Source: CAD feature listing. Evaluate the final solid. Frame: model axes, mm. Coordinates: 2 decimals unless noted, no trailing zeros. Order: outer loops, then holes, each group sorted by start corner. A loop starts at its lowest first (then second) coordinate and runs counter-clockwise, first axis right, second up.
Autodesk Inventor part; units mm, degrees
ref_plane "YZ Plane" through (0, 0, 0) normal (1, 0, 0) x (0, 1, 0)
ref_plane "XZ Plane" through (0, 0, 0) normal (0, 1, 0) x (-1, 0, 0)
ref_plane "XY Plane" through (0, 0, 0) normal (0, 0, 1) x (1, 0, 0)
sketch "Boceto1" plane through (0, 0, 0) normal (0, 0, 1) x (1, 0, 0)
  line L0 (0, 0) -> (0, 210)
  line L1 (0, 210) -> (450, 210)
  line L2 (450, 210) -> (450, 0)
  line L3 (450, 0) -> (0, 0)
  line L4 (0, 210) -> (5, 210)
  line L5 (5, 205) -> (50, 205)
  line L6 (50, 205) -> (50, 202)
  line L7 (5, 205) -> (5, 174.29)
  line L8 (5, 174.29) -> (8, 174.29)
  line L9 (8, 174.29) -> (8, 202)
  line L10 (8, 202) -> (50, 202)
  line L11 (0, 0) -> (5, 0)
  line L12 (0, 0) -> (5, 0)
  line L13 (5, 5) -> (50, 5)
  line L14 (5, 5) -> (5, 35.71)
  line L15 (5, 35.71) -> (8, 35.71)
  line L16 (50, 5) -> (50, 8)
  line L17 (8, 35.71) -> (8, 8)
  line L18 (8, 8) -> (50, 8)
  line L19 (450, 0) -> (445, 0)
  line L20 (445, 5) -> (445, 35.71)
  line L21 (445, 35.71) -> (442, 35.71)
  line L22 (445, 5) -> (400, 5)
  line L23 (400, 5) -> (400, 8)
  line L24 (400, 8) -> (442, 8)
  line L25 (442, 8) -> (442, 35.71)
  line L26 (450, 210) -> (445, 210)
  line L27 (445, 205) -> (400, 205)
  line L28 (445, 205) -> (445, 174.29)
  line L29 (445, 174.29) -> (442, 174.29)
  line L30 (400, 205) -> (400, 202)
  line L31 (400, 202) -> (442, 202)
  line L32 (442, 202) -> (442, 174.29)
  line L33 (5, 63.43) -> (5, 91.14)
  line L34 (5, 91.14) -> (8, 91.14)
  line L35 (8, 91.14) -> (8, 63.43)
  line L36 (8, 63.43) -> (5, 63.43)
  line L37 (5, 118.86) -> (5, 146.57)
  line L38 (5, 118.86) -> (8, 118.86)
  line L39 (8, 118.86) -> (8, 146.57)
  line L40 (8, 146.57) -> (5, 146.57)
  line L41 (445, 63.43) -> (445, 91.14)
  line L42 (445, 63.43) -> (442, 63.43)
  line L43 (442, 63.43) -> (442, 91.14)
  line L44 (442, 91.14) -> (445, 91.14)
  line L45 (445, 118.86) -> (442, 118.86)
  line L46 (442, 118.86) -> (442, 146.57)
  line L47 (442, 146.57) -> (445, 146.57)
  line L48 (445, 146.57) -> (445, 118.86)
  line L49 (350, 205) -> (300, 205)
  line L50 (300, 205) -> (300, 202)
  line L51 (300, 202) -> (350, 202)
  line L52 (350, 202) -> (350, 205)
  line L53 (250, 205) -> (200, 205)
  line L54 (200, 205) -> (200, 202)
  line L55 (200, 202) -> (250, 202)
  line L56 (250, 202) -> (250, 205)
  line L57 (150, 205) -> (100, 205)
  line L58 (100, 205) -> (100, 202)
  line L59 (100, 202) -> (150, 202)
  line L60 (150, 202) -> (150, 205)
  line L61 (350, 8) -> (300, 8)
  line L62 (300, 8) -> (300, 5)
  line L63 (300, 5) -> (350, 5)
  line L64 (350, 5) -> (350, 8)
  line L65 (250, 8) -> (200, 8)
  line L66 (200, 8) -> (200, 5)
  line L67 (200, 5) -> (250, 5)
  line L68 (250, 5) -> (250, 8)
  line L69 (150, 8) -> (100, 8)
  line L70 (100, 8) -> (100, 5)
  line L71 (100, 5) -> (150, 5)
  line L72 (150, 5) -> (150, 8)
  point P0 (450, 30)
  dimension "d8" = 210
  dimension "d9" = 210
  dimension "d10" = 5
  dimension "d11" = 27.72
  dimension "d12" = 5
  dimension "d13" = 5
  dimension "d14" = 450
  dimension "d15" = 5
  dimension "d16" = 5
  dimension "d17" = 5
  dimension "d18" = 45
  dimension "d19" = 30.71
  dimension "d20" = 3
  dimension "d21" = 3
  dimension "d22" = 30.71
  dimension "d23" = 45
  dimension "d24" = 3
  dimension "d25" = 3
  dimension "d26" = 5
  dimension "d27" = 5
  dimension "d29" = 5
  dimension "d30" = 30.71
  dimension "d31" = 45
  dimension "d32" = 5
  dimension "d33" = 3
  dimension "d34" = 3
  dimension "d35" = 5
  dimension "d36" = 5
  dimension "d37" = 45
  dimension "d38" = 30.71
  dimension "d39" = 3
  dimension "d40" = 3
  dimension "d41" = 50
  dimension "d42" = 5
  dimension "d43" = 5
  dimension "d44" = 5
  dimension "d45" = 3
  dimension "d46" = 3
sketch "Boceto2" plane through (0, 0, 0) normal (0, 0, 1) x (1, 0, 0)
  line L0 (449.8604, 0) -> (282.2704, 0)
  circle A0 centre (282.2704, 105) radius 80
  point P0 (0, 0)
extrude "Extrusión1" add sketch "Boceto1" along normal blind 3
extrude "Extrusión2" cut sketch "Boceto2" along normal blind 3
properties part number "Pieza agujero" material "Madera (nogal)"
Q1. Pull-direction query (Y, two-part tool) for faces 1 (the cylindrical face through (358.576, 80.97, 1.479)), 2 (the flat face through (172, 106, 3)); classes: pulls with the +Y half, pulls with the -Y half, needs draft (parallel to the pull), parting line crosses it, or undercut.
Solutions:
face 1: undercut
face 2: needs draft
Q2. Material intervals for line 1 along X through (y, z) = (194, 0.3); line 2 along Y through (x, z) = (405.5, 2.35); line 3 along Y through (x, z) = (247, 2.4), sorted ascending.
Solutions:
line 1: x = 0 to 5, 8 to 442, 445 to 450
line 2: y = 0 to 5, 8 to 202, 205 to 210
line 3: y = 0 to 5, 8 to 33.19, 176.81 to 202, 205 to 210
Q3. Section query A-A on x = 404.5. Output: boundary loops of the cut face in (y, z).
Solutions:
outline: (0, 0) - (5, 0) - (5, 3) - (0, 3) - close; (8, 0) - (202, 0) - (202, 3) - (8, 3) - close; (205, 0) - (210, 0) - (210, 3) - (205, 3) - close
Q4. Section query B-B on y = 105. Output: boundary loops of the cut face in (x, z), plus the area to 3 significant figures.
Solutions:
outline: (0, 0) - (202.27, 0) - (202.27, 3) - (0, 3) - close; (362.27, 0) - (450, 0) - (450, 3) - (362.27, 3) - close
area: 870 mm2
Q5. Section query C-C on y = 126. Output: boundary loops of the cut face in (x, z).
Solutions:
outline: (0, 0) - (5, 0) - (5, 3) - (0, 3) - close; (8, 0) - (205.08, 0) - (205.08, 3) - (8, 3) - close; (359.46, 0) - (442, 0) - (442, 3) - (359.46, 3) - close; (445, 0) - (450, 0) - (450, 3) - (445, 3) - close
Q6. Section query D-D on x = 305.5. Output: boundary loops of the cut face in (y, z), plus the area to 3 significant figures.
Solutions:
outline: (0, 0) - (5, 0) - (5, 3) - (0, 3) - close; (8, 0) - (28.45, 0) - (28.45, 3) - (8, 3) - close; (181.55, 0) - (202, 0) - (202, 3) - (181.55, 3) - close; (205, 0) - (210, 0) - (210, 3) - (205, 3) - close
area: 153 mm2
